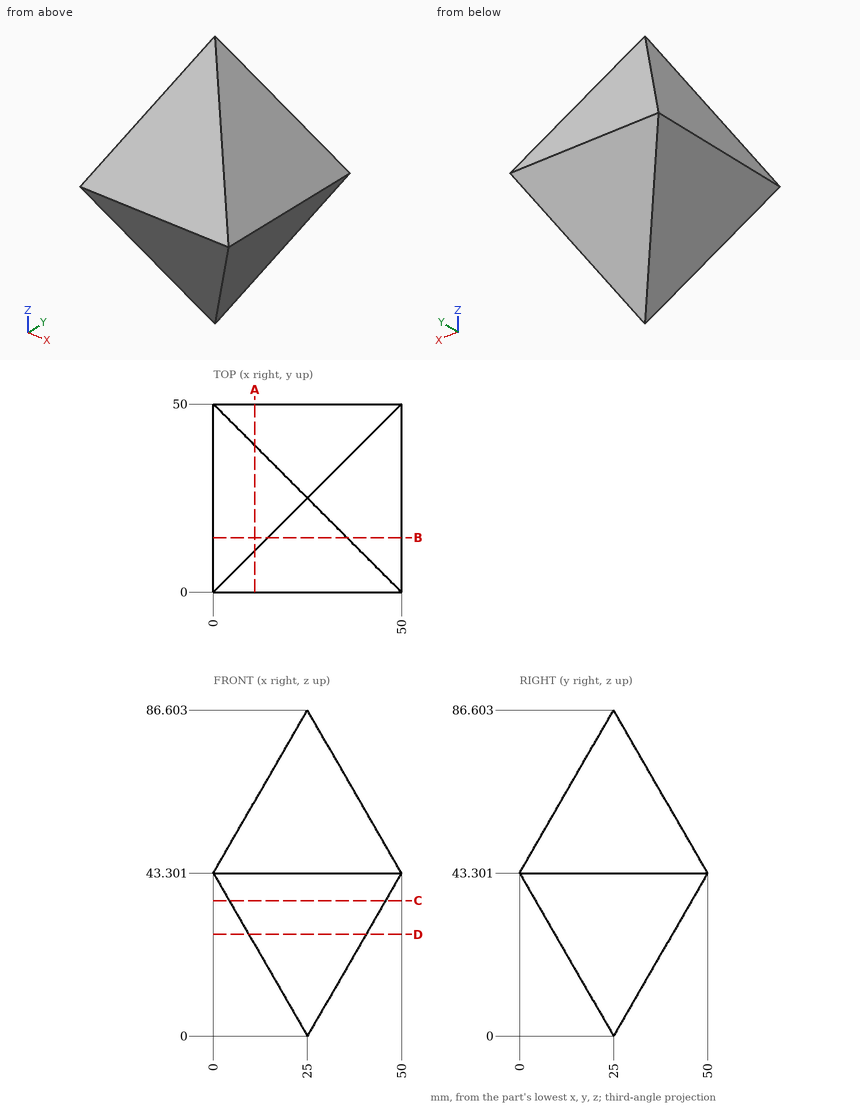
Study the drawing (mm; zero at the part's minimum x, y, z) and answer. Round coordinates to 2 decimals unless told otherwise and drop trailing zeros. Loops run counter-clockwise (first coordinate to the right, second up) from the corner with the lowest first, then second, coordinate; pieces in that order, holes last. Notation, with made-up numbers: (-31.75, 67.5) -> (20.25, 67.5) arc R18 ccw to (20.25, 74.5) -> close; hole circle Ø10 at (25, 65.25). An arc over 180 degrees is marked (long way). Write each question's results on one line, items separated by ' | '. Start each with the question number.
1. Section A-A (x = 11) is taken. Determine the outline of the cut face in (y, z).
2. Section C-C (z = 36) is taken. Determine the outline of the cut face in (x, y) (1 decimal).
3. Find the intervals of material crossed by probe 1 along Z at (x, y) = (42.5, 25.5) (1 decimal); probe 2 along Z at (x, y) = (6.5, 15.5) (1 decimal); probe 3 along Y at (x, z) = (40.5, 31.5) (1 decimal), in increasing order. Write a range as from..to.
4. Section D-D (z = 27) is taken. Determine the outline of the cut face in (x, y).
5. Section B-B (y = 14.5) is taken. Determine the outline of the cut face in (x, z).
6. Given pin 1 Ø1 at (y, z) = (37, 34.5) entering from -X; pin 2 Ø6 at (y, z) = (22, 75.5) entering from +X; pin 3 Ø1 at (x, y) = (22.5, 41) entering from +Z (1 decimal); pin 4 Ø8 at (y, z) = (9, 74) entering from -X, each flat-ended and moving along its own axis, determine where each tip first touches the part or whether it passes through.
Evaluation:
1) outline: (0, 43.3) -> (11, 24.25) -> (39, 24.25) -> (50, 43.3) -> (39, 62.35) -> (11, 62.35) -> close
2) outline: (4.2, 4.2) -> (45.8, 4.2) -> (45.8, 45.8) -> (4.2, 45.8) -> close
3) probe 1: z = 30.3..56.3 | probe 2: z = 32..54.6 | probe 3: y = 6.8..43.2
4) outline: (9.41, 9.41) -> (40.59, 9.41) -> (40.59, 40.59) -> (9.41, 40.59) -> close
5) outline: (0, 43.3) -> (14.5, 18.19) -> (35.5, 18.19) -> (50, 43.3) -> (35.5, 68.42) -> (14.5, 68.42) -> close
6) pin 1: stops at x = 4.79 | pin 2: stops at x = 33.14 | pin 3: stops at z = 59.8 | pin 4: passes through
